The listing builds one solid part. Answer for the finished solid, in the listing's coordinates (mm). Coordinates: 2 decimals unless noted, no trailing zeros. Order: outer loops, then holes, each group sorted by start corner. A loop starts at its lowest first (then second) coordinate and runs counter-clockwise, first axis right, second up.
from build123d import *

# Parameters (mm, degrees)
PAD005_DEPTH    = 2.5
SKETCH012_R     = 1
POCKET003_DEPTH = 3
FILLET001_R     = 0.5


with BuildPart() as part:
    # Sketch008 → Pad005 (new body)
    with BuildSketch(Plane(origin=(43, -2, 9), x_dir=(1, 0, 0), z_dir=(0, 1, 0))):
        with BuildLine():
            Line((71.611134, -34.180398), (57.540096, -23.19394))
            ThreePointArc((56.001794, -20.057013), (56.410347, -21.802308), (57.540096, -23.19394))
            Line((56.001794, -20.057013), (55.961984, -10.029935))
            ThreePointArc((60.498458, -6.050197), (57.324061, -7.007141), (55.961984, -10.029935))
            Line((60.498458, -6.050197), (76.788718, -8.255072))
            Line((76.788718, -8.255072), (71.611134, -34.180398))
        make_face()
    extrude(amount=PAD005_DEPTH)

    # Sketch012 → Pocket003 (cut)
    with BuildSketch(Plane(origin=(43, 0.5, 9), x_dir=(1, 0, 0), z_dir=(0, 1, 0))):
        with Locations((60, -20)):
            Circle(SKETCH012_R)
        with Locations((60, -10)):
            Circle(SKETCH012_R)
    extrude(amount=-POCKET003_DEPTH, mode=Mode.SUBTRACT)

    # Fillet001
    fillet001_edges = [part.edges().sort_by_distance(p)[0] for p in [
        (111.643588, 0.5, 16.152635),
        (100.324061, 0.5, 16.007141),
        (117.199926, 0.5, 30.217735),
        (98.981889, 0.5, 24.043474),
        (107.575615, 0.5, 37.687169),
        (99.410347, 0.5, 30.802308),
        (102, 0.5, 29),
        (102, 0.5, 19),
    ]]
    fillet(fillet001_edges, radius=FILLET001_R)


solid = part.part
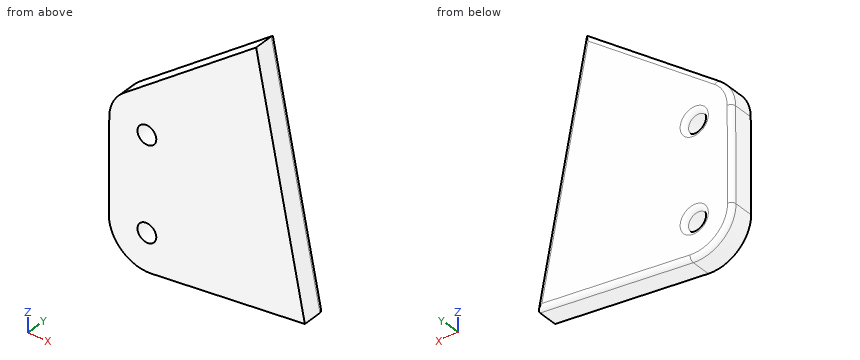
(1) Find section B-B on x = 103. Count the separate pieces of the cut face and the enclosed holes in it, then the cut area to 3 significant figures.
(2) Find section A-A on y = -0.45. Determine the outline of the cut face in (x, z), then the cut area to 3 significant figures.
(3) Find the intervals of material crossed by probe 1 along Z at (x, y) = (103, -1); probe 2 along X at (y, z) = (-0.35, 18.25); probe 3 along X at (y, z) = (-1.15, 29), in increasing order.
Resolved:
1. separate pieces: 3
1. enclosed holes: 0
1. area: 37.4 mm2
2. outline: (98.96, 19.03) arc R4 ccw to (103.5, 15.05) - (119.79, 17.26) - (114.61, 43.18) - (100.54, 32.19) arc R4 ccw to (99, 29.06) - close; hole circle Ø2 at (103, 19); hole circle Ø2 at (103, 29)
2. area: 395 mm2
3. probe 1: z = 15.01 to 18, 20 to 28, 30 to 34.11
3. probe 2: x = 99.04 to 102.34, 103.66 to 119.59
3. probe 3: x = 99 to 102, 104 to 117.44
